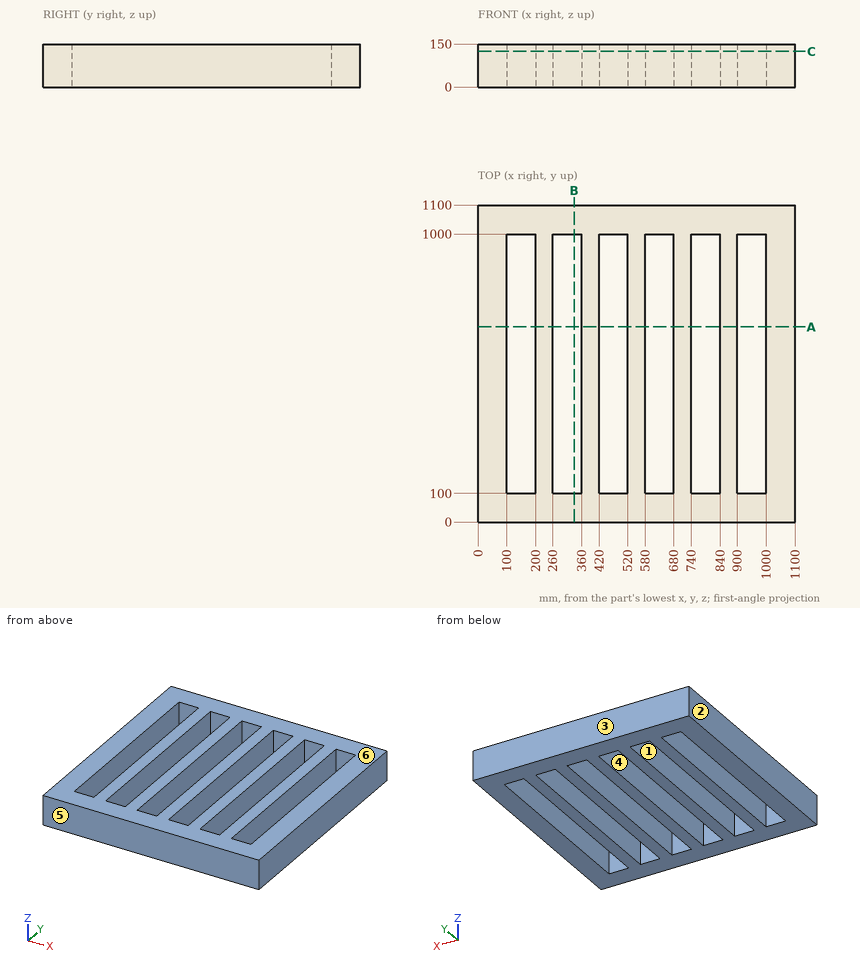
Geometry check sheet. Reference: drawing and pictorial views, mm from the part's lowest x, y, z. A direction names the side the tool comes from. Coordinates: 2 decimals unless noted, no trailing zeros. Loops run counter-clockwise (first coordinate to the right, second up) from the corner with the lowest first, then second, coordinate; pieces in that order, holes last. Notation, with made-up numbers: (-6.75, 27.5) -> (-1.75, 27.5) arc R13 ccw to (-1.75, 51.5) -> close; hole circle Ø1 at (0.5, -22). An arc over 180 degrees is marked (long way). Write item = value, one per line. Start each with the question number.
1. Section check B-B on x = 333.5. Record the cut outline in (y, z).
2. Section check C-C on z = 124. Record the cut outline in (x, y).
3. Tool access check on the marked faces 1 and 2. Record the directions out of +Z, -Z, +X, -X, +Y, -Y that give a thin tool (end or side, any length) a straight path to the whole face; none if there is none.
4. Draft check along Y on the marked faces 3, 4, 5 and 6. Enter one of: released by +Y, released by -Y, zero draft, split by the parting line, or undercut.
5. Material ranges on line 1 (Y direction, x = 643.5, z = 10.5), recorded low to high.
6. Section check A-A on y = 677.5. Record the cut outline in (x, z), then the cut area to 3 significant figures.
Responses:
q1.outline = (0, 0) -> (100, 0) -> (100, 150) -> (0, 150) -> close; (1000, 0) -> (1100, 0) -> (1100, 150) -> (1000, 150) -> close
q2.outline = (0, 0) -> (1100, 0) -> (1100, 1100) -> (0, 1100) -> close; hole (100, 100) -> (200, 100) -> (200, 1000) -> (100, 1000) -> close; hole (260, 100) -> (360, 100) -> (360, 1000) -> (260, 1000) -> close; hole (420, 100) -> (520, 100) -> (520, 1000) -> (420, 1000) -> close; hole (580, 100) -> (680, 100) -> (680, 1000) -> (580, 1000) -> close; hole (740, 100) -> (840, 100) -> (840, 1000) -> (740, 1000) -> close; hole (900, 100) -> (1000, 100) -> (1000, 1000) -> (900, 1000) -> close
q3.face_1 = +Z, -Z
q3.face_2 = +Z, -Z, -X, +Y, -Y
q4.face_3 = released by +Y
q4.face_4 = undercut
q4.face_5 = released by -Y
q4.face_6 = zero draft
q5.line_1 = 0 to 100, 1000 to 1100
q6.outline = (0, 0) -> (100, 0) -> (100, 150) -> (0, 150) -> close; (200, 0) -> (260, 0) -> (260, 150) -> (200, 150) -> close; (360, 0) -> (420, 0) -> (420, 150) -> (360, 150) -> close; (520, 0) -> (580, 0) -> (580, 150) -> (520, 150) -> close; (680, 0) -> (740, 0) -> (740, 150) -> (680, 150) -> close; (840, 0) -> (900, 0) -> (900, 150) -> (840, 150) -> close; (1000, 0) -> (1100, 0) -> (1100, 150) -> (1000, 150) -> close
q6.area = 75,000 mm2
